The drawing under review shows one solid part. Ordinate dimensions are in mm from its lowest x, y, z. Coordinates: 2 decimals unless noted, no trailing zeros. Write each loop counter-clockwise with the first axis right and the second up, starting at its lowest first coordinate (ties: lowest second). Pieces come first, ordered by that corner, then holes.
Q1. To check wall thickness, follow probe 1 along Y at (x, z) = (254, 1447); probe 2 along X at (y, z) = (258, 1241.5); probe 3 along Y at (x, z) = (451.5, 1860.5). State the ranges of each line that lie inside material, in increasing order.
Q2. The part is to be moulded in two halves that separate along Y. For the marked faces 1 and 2, say which applies: +Y half, -Y half, draft (parallel to the pull), parting line (faces both ways), or undercut.
Q3. Add section D-D, the plane z = 1012. Give the boundary of the cut face in (x, y).
Q4. Add section B-B, the plane y = 254. Give the boundary of the cut face in (x, z), plus the area to 3 significant figures.
Q5. Clearance check with flat-ended pins moving along their axes: pin 1 Ø5 at (x, z) = (104, 1361) entering from -Y; pin 2 Ø3 at (x, z) = (139, 316.5) entering from +Y; pin 3 Ø10 at (y, z) = (107.5, 232.5) entering from +X. State where each tip first meets the part, or that it passes through.
Q6. Add section C-C, the plane x = 164.5. Give the boundary of the cut face in (y, z).
Q7. Add section A-A, the plane x = 254. Give the boundary of the cut face in (y, z).
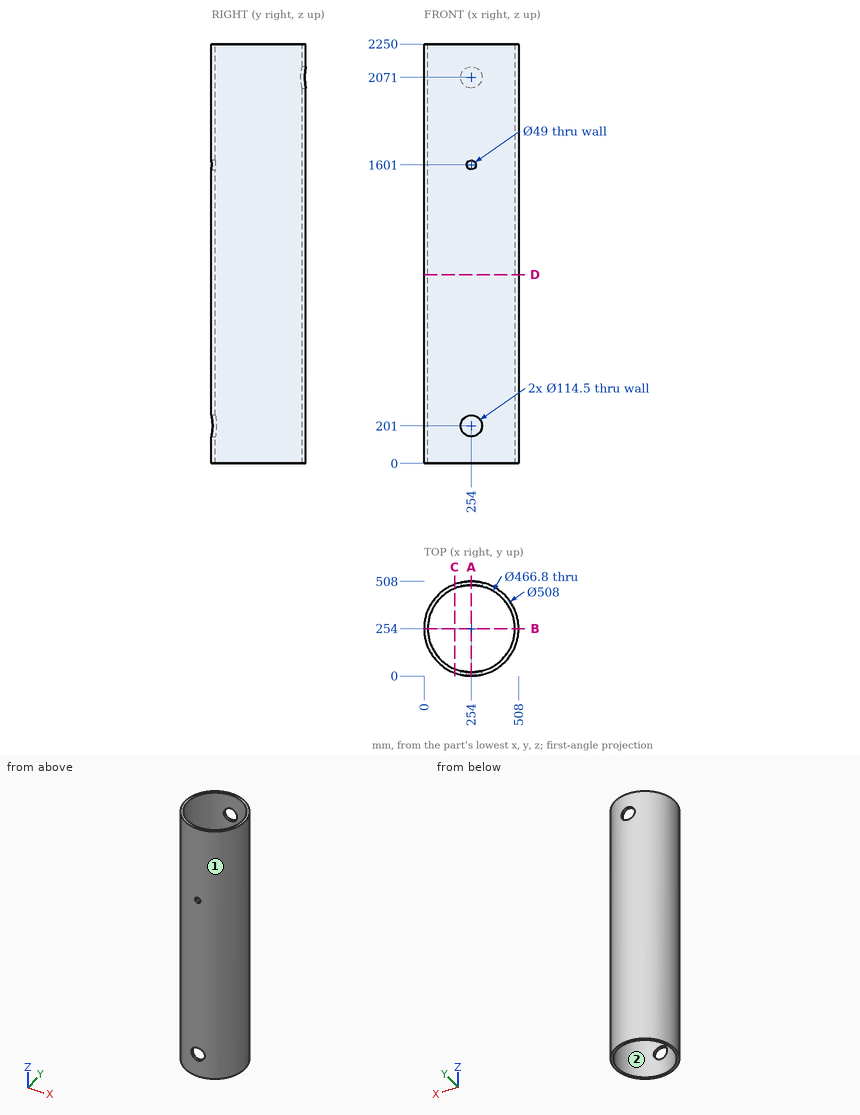
Here are the results:
1. probe 1: y = 0 to 20.6, 487.4 to 508
1. probe 2: x = 0.03 to 20.63, 487.37 to 507.97
1. probe 3: y = 94.28 to 129.62, 378.38 to 413.72
2. face 1: parting line
2. face 2: undercut
3. outline: circle Ø508 at (254, 254); hole circle Ø466.8 at (254, 254)
4. outline: (0, 0) - (20.6, 0) - (20.6, 2250) - (0, 2250) - close; (487.4, 0) - (508, 0) - (508, 2250) - (487.4, 2250) - close
4. area: 92,700 mm2
5. pin 1: stops at y = 47.22
5. pin 2: stops at y = 481.23
5. pin 3: stops at x = 464.94
6. outline: (16.29, 0) - (38.44, 0) - (38.44, 2250) - (16.29, 2250) - close; (469.56, 0) - (491.71, 0) - (491.71, 2250) - (469.56, 2250) - close
7. outline: (0, 0) - (20.6, 0) - (20.6, 143.75) - (0, 143.75) - close; (0, 258.25) - (20.6, 258.25) - (20.6, 1576.5) - (0, 1576.5) - close; (0, 1625.5) - (20.6, 1625.5) - (20.6, 2250) - (0, 2250) - close; (487.4, 0) - (508, 0) - (508, 2013.75) - (487.4, 2013.75) - close; (487.4, 2128.25) - (508, 2128.25) - (508, 2250) - (487.4, 2250) - close
